Read the model definition and answer for the solid it produces. Units are mm, in the model's axes. Face numbers are marked on the shaded views. A direction names the side the tool comes from. Round coordinates to 2 decimals unless told otherwise and drop trailing zeros. Order: outer loops, then holes, each group sorted by start corner. A loop starts at its lowest first (then second) coordinate and runs counter-clockwise, first axis right, second up. Notation, with made-up numbers: (89.25, -29.5) - (126.25, -29.5) arc R12 ccw to (126.25, -22.5) - close; hole circle Ø8 at (74, 80). An arc over 180 degrees is marked (long way). Put each result on its own line as item: value. Start each with the question number.
Q1. This flat-tipped pin is pushed along its axis until it touches: pin 1 Ø1.4 at (x, z) = (2, 1) entering from -Y. Where does it stop, or does it pass through?
Q2. Section D-D on z = -2 is taken. Give the vertices of the cut face in (x, y).
Q3. Section A-A on z = -0.5 is taken. Give the vertices of the cut face in (x, y), then the cut area to 3 significant figures.
Q4. Section B-B on x = 1.75 is taken. Give the vertices of the cut face in (y, z), then the cut area to 3 significant figures.
Q5. Find the intervals of material crossed by line 1 along X through (y, z) = (1.2, 0); line 2 along Y through (x, z) = (0, -2.25), in increasing order. Write a range as from..to.
Q6. Section C-C on y = 1.1 is taken. Give the vertices of the cut face in (x, z), then the cut area to 3 significant figures.
Q7. Which of the six approach directions +Z, -Z, +X, -X, +Y, -Y give full straight-line access (tool end or side, diameter ignored) to the marked faces 1, 2 and 3?
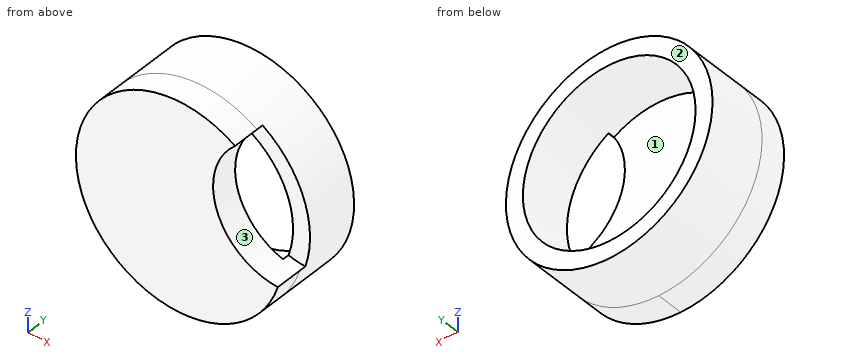
from build123d import *

# Parameters (mm, degrees)
SKETCH_1_R          = 3.05
SKETCH_1_R_2        = 2.55
EXTRUDE_1_DEPTH     = 1.8
EXTRUDE_START       = 0.8
SKETCH_2_R          = 3.05
EXTRUDE_2_DEPTH     = 0.8
SKETCH_3_R          = 2
CUT_EXTRUDE_1_DEPTH = 1


with BuildPart() as part:
    # 草图1 → 凸台-拉伸1 (new body)
    with BuildSketch(Plane(origin=(0, 0, 0), x_dir=(1, 0, 0), z_dir=(0, 1, 0))):
        with Locations(Location((0, 0, 0), (0, 0, 270))):
            Circle(SKETCH_1_R)
        with Locations(Location((0, 0, 0), (0, 0, 270))):
            Circle(SKETCH_1_R_2, mode=Mode.SUBTRACT)
    extrude(amount=EXTRUDE_1_DEPTH)

    # 草图2 → 凸台-拉伸2 (add)
    with BuildSketch(Plane.XZ.offset(EXTRUDE_START)):
        with Locations(Location((0, 0, 0), (0, 0, 270))):
            Circle(SKETCH_2_R)
    extrude(amount=-EXTRUDE_2_DEPTH)

    # 草图3 → 切除-拉伸1 (cut)
    with BuildSketch(Plane.XZ.offset(0.8)):
        with Locations((3, 1.092527685)):
            Circle(SKETCH_3_R)
    extrude(amount=-CUT_EXTRUDE_1_DEPTH, mode=Mode.SUBTRACT)


solid = part.part
Findings:
1. pin 1: y = 0.2
2. outline: (-2.3, -0.8) - (2.3, -0.8) - (2.3, 1.8) - (1.58, 1.8) - (1.58, 0) - (-1.58, 0) - (-1.58, 1.8) - (-2.3, 1.8) - close
3. outline: (-3.01, -0.8) - (1.79, -0.8) - (1.79, 0) - (-2.5, 0) - (-2.5, 1.8) - (-3.01, 1.8) - close; (2.5, 0.2) - (3.01, 0.2) - (3.01, 1.8) - (2.5, 1.8) - close
3. area: 5.57 mm2
4. outline: (-0.8, -2.5) - (1.8, -2.5) - (1.8, -1.85) - (0, -1.85) - (0, -0.47) - (-0.8, -0.47) - close; (0.2, 1.85) - (1.8, 1.85) - (1.8, 2.5) - (0.2, 2.5) - close
4. area: 3.81 mm2
5. line 1: -3.05..-2.55, 2.55..3.05
5. line 2: -0.8..0
6. outline: circle Ø6.1 at (0, 0); hole circle Ø5.1 at (0, 0)
6. area: 8.80 mm2
7. face 1: +Y
7. face 2: +Z, -Z, +X, -X, +Y
7. face 3: +X, -Y
